Here's how the part is built. I have some questions about the finished solid (model axes, mm). Round coordinates to 2 decimals unless told otherwise and drop trailing zeros. Order: outer loops, then holes, each group sorted by start corner. A loop starts at its lowest first (then second) coordinate and runs counter-clockwise, first axis right, second up. Notation, with made-up numbers: M 53,-28.5 L 72,-28.5 A10 ccw 72,-10.5 Z; hole C -28.75,81.5 d9. An arc over 180 degrees is marked long. Write each question's results on one line, items separated by ' | '. Start each with the question number.
```python
from build123d import *

# Parameters (mm, degrees)
SKETCH2_R             = 1.7
BOSS_EXTRUDE3_DEPTH   = 1.5
FILLET4_R             = 5
BODY_MOVE_COPY1_ANGLE = 91.5
BODY_MOVE_COPY2_ANGLE = 180
SKETCH3_W             = 14
SKETCH3_H             = 14
CUT_EXTRUDE6_DEPTH    = 10


with BuildPart() as part:
    # Sketch2 → Boss-Extrude3 (new body)
    with BuildSketch(Plane(origin=(0, 0, 0), x_dir=(1, 0, 0), z_dir=(0, 1, 0))):
        Polygon((41.198193182, -31.056403409), (41.198193182, 53.223596591), (7.648193182, 53.223596591), (7.648193182, 22.223596591), (-10.851806818, 22.223596591), (-10.851806818, 53.223596591), (-40.691806818, 53.223596591), (-40.691806818, -31.056403409), align=None)
        with Locations(Location((-35.691806818, -26.056403409, 0), (0, 0, 270))):
            Circle(SKETCH2_R, mode=Mode.SUBTRACT)
        with Locations(Location((36.198193182, -26.056403409, 0), (0, 0, 270))):
            Circle(SKETCH2_R, mode=Mode.SUBTRACT)
        with Locations(Location((-35.691806818, 48.223596591, 0), (0, 0, 270))):
            Circle(SKETCH2_R, mode=Mode.SUBTRACT)
        with Locations(Location((36.198193182, 48.223596591, 0), (0, 0, 270))):
            Circle(SKETCH2_R, mode=Mode.SUBTRACT)
    extrude(amount=BOSS_EXTRUDE3_DEPTH)

    # Fillet4
    fillet4_edges = [part.edges().sort_by_distance(p)[0] for p in [
        (41.198193182, 0.75, -53.223596591),
        (41.198193182, 0.75, 31.056403409),
        (-40.691806818, 0.75, 31.056403409),
        (-40.691806818, 0.75, -53.223596591),
    ]]
    fillet(fillet4_edges, radius=FILLET4_R)


with BuildPart() as part_1:
    # Body-Move_Copy1: moved
    add(part.part.rotate(Axis((0, 0.75, -12.283596591), (-1, 0, 0)), BODY_MOVE_COPY1_ANGLE))


with BuildPart() as part_2:
    # Body-Move_Copy2: moved
    add(part_1.part.rotate(Axis((0.403193182, 0.75, 0), (0, 0, 1)), BODY_MOVE_COPY2_ANGLE))

    # Sketch3 → Cut-Extrude6 (cut)
    with BuildSketch(Plane(origin=(0, 0.341583523, -13.044548447), x_dir=(-1, 0, 0), z_dir=(-2.1436792936287095e-13, 0.026176948305881326, -0.9996573249756094))):
        with Locations((-19.598193182, -20.81180408)):
            Rectangle(SKETCH3_W, SKETCH3_H)
        with Locations((-0.548193182, -20.81180408)):
            Rectangle(SKETCH3_W, SKETCH3_H)
        with Locations((18.501806818, -20.81180408)):
            Rectangle(SKETCH3_W, SKETCH3_H)
        with Locations((-0.548193182, -1.76180408)):
            Rectangle(SKETCH3_W, SKETCH3_H)
    extrude(amount=-CUT_EXTRUDE6_DEPTH, mode=Mode.SUBTRACT)


solid = part_2.part
```
(1) If we mould it in two halves opening along Y, with no side actions, what happens to faces 1 (the flat face through (26.598, -21, -13)), 2 (the cylindrical face through (-38.97, -41.07, -13.39)), 3 (the flat face through (11.658, 26, -12))? For each: pulls with the +Y half, pulls with the -Y half, needs draft (parallel to the pull), parting line crosses it, or undercut.
(2) I want a section at D-D on y = -17. Write out the boundary of the cut face in (x, z), and give its area (3 significant figures).
(3) Please list where these lines run through material, in increasing order: line 1 (X direction, y = -23, z = -13.4); line 2 (X direction, y = 14, z = -11.3); line 3 (Z direction, x = -8.5, y = 10.5).
(4) I want a section at B-B on x = 4.5. Write out the boundary of the cut face in (y, z).
(5) I want a section at A-A on x = 22. Write out the boundary of the cut face in (y, z).
(6) I'm going to push flat-ended pins straight in: pin 1 Ø1.5 at (x, y) = (11, -1) entering from +Z; pin 2 Ø1.5 at (x, z) = (13, -11) entering from +Y. Where does each tip first touch, or does it pass through?
(7) I want a section at C-C on y = 32.5. Write out the boundary of the cut face in (x, z), and give its area (3 significant figures).
Solutions:
1) face 1: undercut | face 2: pulls with the -Y half | face 3: needs draft
2) outline: M -40.39,-13.5 L -25.5,-13.5 L -25.5,-12 L -40.39,-12 Z; M -11.5,-13.5 L -6.45,-13.5 L -6.45,-12 L -11.5,-12 Z; M 7.55,-13.5 L 12.6,-13.5 L 12.6,-12 L 7.55,-12 Z; M 26.6,-13.5 L 41.5,-13.5 L 41.5,-12 L 26.6,-12 Z | area: 59.9 mm^2
3) line 1: -40.39 to -25.5, -11.5 to -6.45, 7.55 to 12.6, 26.6 to 41.5 | line 2: -40.39 to -6.84, 11.66 to 41.5 | line 3: -12.78 to -11.28
4) outline: M -42.59,-12.67 L -42.56,-14.17 L -27.46,-13.77 L -27.5,-12.27 Z; M -13.5,-11.91 L -13.47,-13.41 L -8.42,-13.27 L -8.46,-11.77 Z; M 5.54,-11.41 L 5.58,-12.91 L 10.71,-12.77 L 10.67,-11.27 Z
5) outline: M -42.59,-12.67 L -42.56,-14.17 L -27.46,-13.77 L -27.5,-12.27 Z; M -13.5,-11.91 L -13.47,-13.41 L 41.7,-11.96 L 41.66,-10.46 Z
6) pin 1: z = -11.56 | pin 2: y = 41.69
7) outline: M -40.39,-12.2 L -6.84,-12.2 L -6.84,-10.7 L -40.39,-10.7 Z; M 11.66,-12.2 L 41.5,-12.2 L 41.5,-10.7 L 11.66,-10.7 Z | area: 95.1 mm^2
